Could you check a few things on this model? Use its own coordinates, in mm. A direction names the side the tool comes from. Give positions to 0.01 mm unless a question says otherwise; leave off trailing zeros. Write each loop counter-clockwise with the first axis right and the second up, starting at its lowest first coordinate (ties: lowest second). Pieces come first, ordered by that corner, then holes. Notation, with made-up numbers: (70.25, 65) -> (112.25, 65) arc R29 ccw to (112.25, 101) -> close; hole circle Ø3 at (-12.75, -30). An arc over 180 degrees is marked (long way). One line per question, with ' | ' between items.
from build123d import *
from build123d.topology import SkipClean

# Parameters (mm, degrees)
BOSS_EXTRUDE1_DEPTH   = 5
MIRROR1_START         = -33
MIRROR1_OUTLINE_W     = 146
MIRROR1_OUTLINE_H     = 5
MIRROR1_DEPTH         = 66
MIRROR1_START_2       = -38
MIRROR1_2_OUTLINE_W   = 27.4
MIRROR1_2_OUTLINE_H   = 5
MIRROR1_2_OUTLINE_W_2 = 30.4
MIRROR1_2_DEPTH       = 76
MIRROR1_START_3       = 12.666666667
MIRROR1_3_OUTLINE_W   = 3
MIRROR1_3_OUTLINE_H   = 5
MIRROR1_3_DEPTH       = 25.333333333
MIRROR1_4_OUTLINE_W   = 3
MIRROR1_4_OUTLINE_H   = 5
MIRROR1_4_DEPTH       = 25.333333333
CUT_EXTRUDE1_DEPTH    = 86.117565755
SKETCH3_R             = 1.6
CUT_EXTRUDE2_DEPTH    = 86.117565755
CHAMFER1_SIZE         = 1.5


# Read off the part's stored shape, not the designer's step: Mirror1
with BuildPart() as part:
    # Sketch1 → Boss-Extrude1 (new body)
    with BuildSketch(Plane(origin=(0, 0, 0), x_dir=(1, 0, 0), z_dir=(0, 1, 0))):
        Polygon((-76, 38), (-76, 12.666666667), (-73, 12.666666667), (-73, 0), (0, 0), (0, 38), (-15.2, 38), (-15.2, 33), (-45.6, 33), (-45.6, 38), align=None)
    extrude(amount=BOSS_EXTRUDE1_DEPTH)

    # Mirror1 outline → Mirror1 (add)
    with BuildSketch(Plane.XY.offset(MIRROR1_START)):
        with Locations((0, 2.5)):
            Rectangle(MIRROR1_OUTLINE_W, MIRROR1_OUTLINE_H)
    extrude(amount=MIRROR1_DEPTH)

    # Mirror1 2 outline → Mirror1 2 (add)
    with BuildSketch(Plane.XY.offset(MIRROR1_START_2)):
        with Locations((-59.3, 2.5)):
            Rectangle(MIRROR1_2_OUTLINE_W, MIRROR1_2_OUTLINE_H)
        with Locations((0, 2.5)):
            Rectangle(MIRROR1_2_OUTLINE_W_2, MIRROR1_2_OUTLINE_H)
        with Locations((59.3, 2.5)):
            Rectangle(MIRROR1_2_OUTLINE_W, MIRROR1_2_OUTLINE_H)
    extrude(amount=MIRROR1_2_DEPTH)

    # Mirror1 3 outline → Mirror1 3 (add)
    with BuildSketch(Plane.XY.offset(MIRROR1_START_3)):
        with Locations((-74.5, 2.5)):
            Rectangle(MIRROR1_3_OUTLINE_W, MIRROR1_3_OUTLINE_H)
        with Locations((74.5, 2.5)):
            Rectangle(MIRROR1_3_OUTLINE_W, MIRROR1_3_OUTLINE_H)
    extrude(amount=MIRROR1_3_DEPTH)

    # Mirror1 4 outline → Mirror1 4 (add)
    with BuildSketch(Plane.XY.offset(MIRROR1_START_2)):
        with Locations((74.5, 2.5)):
            Rectangle(MIRROR1_4_OUTLINE_W, MIRROR1_4_OUTLINE_H)
    extrude(amount=MIRROR1_4_DEPTH)

    # Sketch2 → Cut-Extrude1 (cut, through all)
    with BuildSketch(Plane(origin=(0, 5, 0), x_dir=(1, 0, 0), z_dir=(0, 1, 0))):
        with BuildLine():
            Line((0, 18), (0, -18))
            ThreePointArc((0, -18), (-18, 0), (0, 18))
        make_face()
        with BuildLine():
            ThreePointArc((-19.342622189, 16.230387145), (-19.835649522, 21.865715356), (-25.470977734, 21.372688022))
            ThreePointArc((-25.470977734, 21.372688022), (-33.25, 0), (-25.470977734, -21.372688022))
            ThreePointArc((-25.470977734, -21.372688022), (-19.835649522, -21.865715356), (-19.342622189, -16.230387145))
            ThreePointArc((-19.342622189, -16.230387145), (-25.25, 0), (-19.342622189, 16.230387145))
        make_face()
    cut_extrude1 = extrude(amount=-CUT_EXTRUDE1_DEPTH, mode=Mode.SUBTRACT)

    # Sketch3 → Cut-Extrude2 (cut, through all)
    with BuildSketch(Plane(origin=(0, 5, 0), x_dir=(1, 0, 0), z_dir=(0, 1, 0))):
        with Locations(Location((-42.5, 0, 0), (0, 0, 270))):
            Circle(SKETCH3_R)
        with Locations(Location((42.5, 0, 0), (0, 0, 270))):
            Circle(SKETCH3_R)
    extrude(amount=-CUT_EXTRUDE2_DEPTH, mode=Mode.SUBTRACT)

    # Chamfer1
    chamfer1_edges = [part.edges().sort_by_distance(p)[0] for p in [
        (-42.5, 5, -1.6),
        (42.5, 5, -1.6),
    ]]
    chamfer(chamfer1_edges, length=CHAMFER1_SIZE)

    # Mirror3: Cut-Extrude1 across plane
    with SkipClean():  # the faces are left unmerged after this step: merging them gives an invalid solid
        add(cut_extrude1.mirror(Plane(origin=(0, 0, 0), x_dir=(0, 0, 1), z_dir=(1, 0, 0))), mode=Mode.SUBTRACT)


solid = part.part
Q1. Imagine slicing it at B-B on z = 0. Please give me the cut outline in (x, y), and give its area (4 significant figures).
Answer below:
outline: (-73, 0) -> (-44.1, 0) -> (-44.1, 3.5) -> (-45.6, 5) -> (-73, 5) -> close; (-40.9, 0) -> (-33.25, 0) -> (-33.25, 5) -> (-39.4, 5) -> (-40.9, 3.5) -> close; (-25.25, 0) -> (-18, 0) -> (-18, 5) -> (-25.25, 5) -> close; (18, 0) -> (25.25, 0) -> (25.25, 5) -> (18, 5) -> close; (33.25, 0) -> (40.9, 0) -> (40.9, 3.5) -> (39.4, 5) -> (33.25, 5) -> close; (44.1, 0) -> (73, 0) -> (73, 5) -> (45.6, 5) -> (44.1, 3.5) -> close | area: 433.5 mm^2
Q2. If we mould it in two halves opening along X, with no side actions, what happens to faces 1 (the flat face through (-61, 2, -38)), 2 (the cylindrical face through (25.25, 2.54, 0.25)), 3 (the flat face through (73, 2, 0))? For each: +X half, -X half, draft (parallel to the pull), parting line (faces both ways), or undercut.
Answer below:
face 1: draft | face 2: undercut | face 3: +X half
Q3. If I drill on line 1 along X through (y, z) = (2.3, 0); line 2 along Z through (x, y) = (0, 2.65); line 3 along X through (y, z) = (2.35, 4.5), over which ranges is the centre line in solid material (lowest first)?
Answer below:
line 1: x = -73 to -44.1, -40.9 to -33.25, -25.25 to -18, 18 to 25.25, 33.25 to 40.9, 44.1 to 73 | line 2: z = -38 to -18, 18 to 38 | line 3: x = -73 to -32.94, -24.85 to -17.43, 17.43 to 24.85, 32.94 to 73
Q4. Will these pins go through, and if not, where does the flat tip stop? pin 1 (2.5 mm diameter, centred on y = 3.5, z = 5.5, fed in from -X); pin 2 (21.5 mm diameter, centred on x = 0, z = 0, fed in from +Y); pin 3 (2.5 mm diameter, centred on x = 27, y = 2, fed in from -Z).
Answer below:
pin 1: stops at x = -73 | pin 2: passes through | pin 3: stops at z = -33
Q5. Imagine slicing it at A-A on x = 0. Please give me the cut outline in (y, z).
Answer below:
outline: (0, -38) -> (5, -38) -> (5, -18) -> (0, -18) -> close; (0, 18) -> (5, 18) -> (5, 38) -> (0, 38) -> close
Q6. Imagine slicing it at C-C on x = -42.5. Please give me the cut outline in (y, z).
Answer below:
outline: (0, -33) -> (5, -33) -> (5, -3.1) -> (3.5, -1.6) -> (0, -1.6) -> close; (0, 1.6) -> (3.5, 1.6) -> (5, 3.1) -> (5, 33) -> (0, 33) -> close
Q7. Imagine slicing it at D-D on y = 1. Count the separate pieces of the cut face and the enclosed holes in it, and give its area (3 significant figures).
Answer below:
separate pieces: 1 | enclosed holes: 5 | area: 9,000 mm^2
Q8. On a 3-axis mill with a long thin cutter (end or side, diameter ignored), from which of +Z, -Z, +X, -X, +Y, -Y can I reach the whole of each face in a straight line? I mean faces 4 (the cylindrical face through (33.25, 2.54, -0.32)), 5 (the flat face through (74, 3, 12.667)), 6 (the flat face through (-15.2, 2, -36)), 7 (the flat face through (-75, 2, -12.667)). Say none if no direction works.
Answer below:
face 4: +Y, -Y | face 5: +X, +Y, -Y | face 6: -Z, +Y, -Y | face 7: -X, +Y, -Y
